Model file for the job. Use its own axes, mm. Face numbers are marked on the shaded views. Give positions to 0.01 mm unless a question says otherwise; leave off trailing zeros. Write each loop counter-clockwise with the first axis right and the second up, starting at its lowest first coordinate (ties: lowest second). Pieces come first, ordered by that corner, then holes. Notation, with made-up numbers: (76.5, 89) - (132.5, 89) arc R8 cw to (132.5, 104) - close; hole circle Ø6 at (79.5, 33). An arc over 180 degrees is marked (long way). One line per item, written item: value. Start each with the question number.
(1) Probe L1, parallel to Z at x = -3.5, y = -2.5; L2, parallel to Z at x = 3.25, y = -11.5; L3, parallel to Z at x = 0, y = -10. List the from-to ranges inside material, lowest first.
(2) Drop flat-ended pins along their axis: P1, Ø3, axis at y = -3.5, z = -16, coming from the +X side (3 decimals); P2, Ø2, axis at x = 9, y = -6.5, coming from the -Z side; P3, Ø1.5, axis at y = -3.5, z = -21.5, coming from the +X side. Give the stop position or say it passes through.
(3) Cut at B-B, the plane x = 0. List the corners of the cut face in (y, z), and give its area (3 significant figures).
(4) Cut at C-C, the plane z = -20. List the corners of the cut face in (x, y).
(5) Mould opens along Y. For the marked faces 1, 2 and 3 say: pulls with the +Y half, pulls with the -Y half, needs draft (parallel to the pull), parting line crosses it, or undercut.
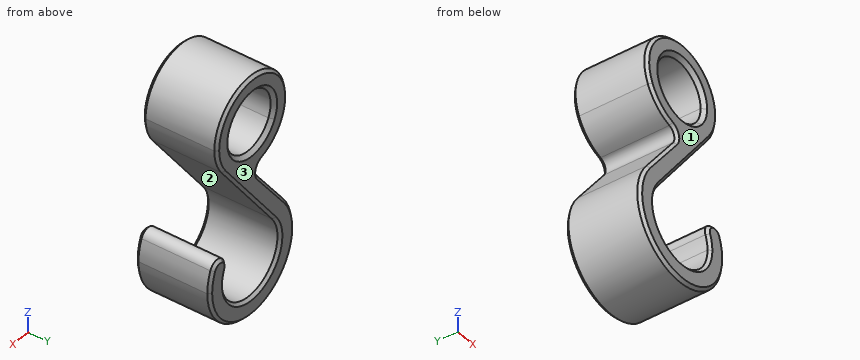
from build123d import *

# Parameters (mm, degrees)
F1_DEPTH = 16
F2_R     = 1.99999
F3_SIZE  = 0.8
F4_SIZE  = 0.6


# Not quite as in the source:
# - a fillet or chamfer is up to 0.001 mm smaller than in the source, because OpenCascade refuses the exact size


with BuildPart() as f1:
    # F0 (on Front) → F1 (new body)
    with BuildSketch(Plane.XZ):
        with BuildLine():
            ThreePointArc((6.3, 0), (5.9640762947, -2.0297275557), (4.9921289046, -3.843))
            Line((4.9921289046, -3.843), (0.2548985956, -9.9967508074))
            ThreePointArc((0.2548985956, -9.9967508074), (4.5857760478, -8.8865436498), (8, -6))
            ThreePointArc((8, -6), (9.4868329805, -3.1622776602), (10, 0))
            ThreePointArc((10, 0), (-2.2360679775, 9.7467943448), (-9, -4.3588989435))
            Line((-9, -4.3588989435), (-5.67, -2.7461063344))
            ThreePointArc((-5.67, -2.7461063344), (-1.4087228258, 6.1404804372), (6.3, 0))
        make_face()
        with BuildLine():
            ThreePointArc((8, -6), (4.5857760478, -8.8865436498), (0.2548985956, -9.9967508074))
            Line((0.2548985956, -9.9967508074), (-9.5088169611, -22.68))
            ThreePointArc((-9.5088169611, -22.68), (-5.7581726954, -19.4717785353), (-1.033436854, -18.044582472))
            Line((-1.033436854, -18.044582472), (8, -6))
        make_face()
        with BuildLine():
            ThreePointArc((-1.033436854, -18.044582472), (-5.7581726954, -19.4717785353), (-9.5088169611, -22.68))
            ThreePointArc((-9.5088169611, -22.68), (-3.8661477252, -41.3601453233), (12, -30))
            ThreePointArc((12, -30), (11.4891252931, -26.5358983849), (10, -23.3667504193))
            Line((10, -23.3667504193), (6.6666666667, -25.5778336129))
            ThreePointArc((6.6666666667, -25.5778336129), (7.6594168621, -27.6905989232), (8, -30))
            ThreePointArc((8, -30), (-2.5298221281, -37.5894663844), (-6.4, -25.2))
            Line((-6.4, -25.2), (-1.033436854, -18.044582472))
        make_face()
        with BuildLine():
            Line((0.2548985956, -9.9967508074), (4.9921289046, -3.843))
            ThreePointArc((4.9921289046, -3.843), (-0.6447257044, -6.2669233892), (-5.67, -2.7461063344))
            Line((-5.67, -2.7461063344), (-9, -4.3588989435))
            ThreePointArc((-9, -4.3588989435), (-5.202455483, -8.5401672669), (0.2548985956, -9.9967508074))
        make_face()
    extrude(amount=F1_DEPTH)

    # F2 (radius 2 in the source; OpenCascade refuses exactly that, so slightly less here)
    f2_edges = [f1.edges().sort_by_distance(p)[0] for p in [
        (4.992129, -8, -3.843),
        (8, -8, -6),
        (10, -8, -23.36675),
        (6.666667, -8, -25.577834),
        (0.254899, -8, -9.996751),
    ]]
    fillet(f2_edges, radius=F2_R)

    # F3
    f3_edges = [f1.edges().sort_by_distance(p)[0] for p in [
        (-4.992129, -16, 3.843),
        (-4.992129, 0, 3.843),
    ]]
    chamfer(f3_edges, length=F3_SIZE)

    # F4
    f4_edges = [f1.edges().sort_by_distance(p)[0] for p in [
        (-3.134832, -16, 9.495937),
        (0.8, 0, -15.6),
        (-5.675293, 0, -17.70018),
        (-1.523485, 0, -10.885342),
        (-1.625379, 0, -41.889413),
        (-3.134832, 0, 9.495937),
        (9.862297, 0, -24.340194),
        (8.164968, 0, -24.583973),
        (-1.033792, 0, -37.932923),
        (7.360063, 0, -25.658852),
        (-5.675293, -16, -17.70018),
        (-1.523485, -16, -10.885342),
        (-1.625379, -16, -41.889413),
        (9.862297, -16, -24.340194),
        (0.8, -16, -15.6),
        (8.164968, -16, -24.583973),
        (-1.033792, -16, -37.932923),
        (7.360063, -16, -25.658852),
    ]]
    chamfer(f4_edges, length=F4_SIZE)


solid = f1.part
Answers follow:
1. L1: z = -41.48 to -37.19, -21.33 to -14.87, -9.37 to -5.24, 5.24 to 9.37
1. L2: z = -41.55 to -37.31, -12.33 to -5.4, 5.4 to 9.46
1. L3: z = -42 to -38, -16.67 to -6.3, 6.3 to 10
2. P1: stops at x = 1.625
2. P2: stops at z = -38.94
2. P3: stops at x = -3.06
3. outline: (-16, -41.4) - (-15.4, -42) - (-0.6, -42) - (0, -41.4) - (0, -38.6) - (-0.6, -38) - (-15.4, -38) - (-16, -38.6) - close; (-16, -15.67) - (-15.4, -16.67) - (-0.6, -16.67) - (0, -15.67) - (0, -7.1) - (-0.8, -6.3) - (-15.2, -6.3) - (-16, -7.1) - close; (-16, 7.1) - (-15.2, 6.3) - (-0.8, 6.3) - (0, 7.1) - (0, 9.4) - (-0.6, 10) - (-15.4, 10) - (-16, 9.4) - close
3. area: 286 mm²
4. outline: (-7.45, -15.4) - (-6.69, -16) - (-3.25, -16) - (-2.5, -15.4) - (-2.5, -0.6) - (-3.25, 0) - (-6.69, 0) - (-7.45, -0.6) - close
5. face 1: pulls with the -Y half
5. face 2: needs draft
5. face 3: pulls with the +Y half
